```python
from build123d import *

# Parameters (mm, degrees)
SKETCH1_W           = 150
SKETCH1_H           = 30
BOSS_EXTRUDE1_DEPTH = 15
CUT_EXTRUDE1_DEPTH  = 5
SKETCH3_R           = 0.75
CUT_EXTRUDE2_DEPTH  = 30
CUT_EXTRUDE3_DEPTH  = 5


with BuildPart() as part:
    # Sketch1 → Boss-Extrude1 (new body)
    with BuildSketch(Plane(origin=(0, 0, 0), x_dir=(1, 0, 0), z_dir=(0, 1, 0))):
        with Locations((75, 15)):
            Rectangle(SKETCH1_W, SKETCH1_H)
    extrude(amount=BOSS_EXTRUDE1_DEPTH)

    # Sketch2 → Cut-Extrude1 (cut)
    with BuildSketch(Plane(origin=(0, 15, 0), x_dir=(1, 0, 0), z_dir=(0, 1, 0))):
        with BuildLine():
            Line((-20, 22.5), (20, 22.5))
            ThreePointArc((20, 22.5), (27.5, 15), (20, 7.5))
            Line((20, 7.5), (-20, 7.5))
            ThreePointArc((-20, 7.5), (-27.5, 15), (-20, 22.5))
        make_face()
        with BuildLine():
            Line((170, 22.5), (130, 22.5))
            ThreePointArc((130, 22.5), (122.5, 15), (130, 7.5))
            Line((130, 7.5), (170, 7.5))
            ThreePointArc((170, 7.5), (177.5, 15), (170, 22.5))
        make_face()
    extrude(amount=-CUT_EXTRUDE1_DEPTH, mode=Mode.SUBTRACT)

    # Sketch3 → Cut-Extrude2 (cut)
    with BuildSketch(Plane.XY):
        with Locations((25, 7.5)):
            Circle(SKETCH3_R)
        with Locations((75, 7.5)):
            Circle(SKETCH3_R)
        with Locations((125, 7.5)):
            Circle(SKETCH3_R)
    extrude(amount=-CUT_EXTRUDE2_DEPTH, mode=Mode.SUBTRACT)

    # Sketch4 → Cut-Extrude3 (cut)
    with BuildSketch(Plane(origin=(0, 15, 0), x_dir=(1, 0, 0), z_dir=(0, 1, 0))):
        with BuildLine():
            Line((37.5, 25), (112.5, 25))
            ThreePointArc((112.5, 25), (116.035533906, 23.535533906), (117.5, 20))
            Line((117.5, 20), (117.5, 10))
            ThreePointArc((117.5, 10), (116.035533906, 6.464466094), (112.5, 5))
            Line((112.5, 5), (37.5, 5))
            ThreePointArc((37.5, 5), (33.964466094, 6.464466094), (32.5, 10))
            Line((32.5, 10), (32.5, 20))
            ThreePointArc((32.5, 20), (33.964466094, 23.535533906), (37.5, 25))
        make_face()
    extrude(amount=-CUT_EXTRUDE3_DEPTH, mode=Mode.SUBTRACT)


solid = part.part
```
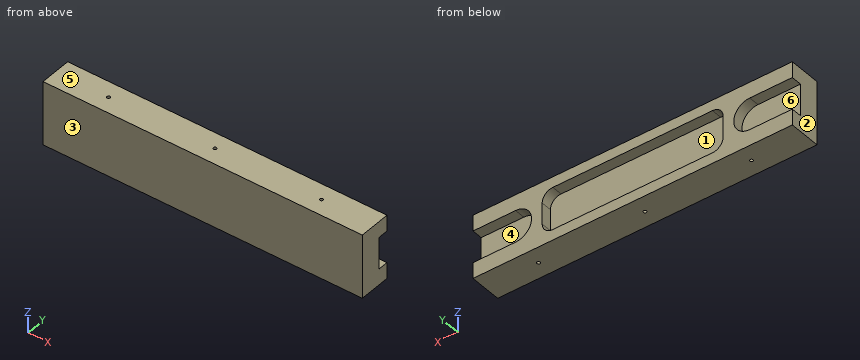
Verification items for the finished model (mm, model axes). Face numbers are marked on the shaded views. A direction names the side the tool comes from. Coordinates: 2 decimals unless noted, no trailing zeros. Write each loop counter-clockwise with the first axis right and the second up, starting at its lowest first coordinate (ties: lowest second). Pieces come first, ordered by that corner, then holes. Notation, with made-up numbers: M 20.25,31 L 72.25,31 A7 cw 72.25,38 Z; hole C 53,17.25 d11. An arc over 180 degrees is marked long. One line per item, written item: value.
Item 1: Access from +Z, -Z, +X, -X, +Y, -Y to the whole of each face (thin tool, end or side, straight path). Record for the marked faces 4, 5 and 6.
Check sheet entries:
face 4: +X, +Y
face 5: +Z, +X, -X, +Y, -Y
face 6: -X, +Y
Item 2: Scan lines: line 1 along Y through (x, z) = (25, -21.25); line 2 along X through (y, z) = (7.25, -22); line 3 along Y through (x, z) = (75, -16.75). Record each from-to range of solid material in increasing order.
Check sheet entries:
line 1: y = 0 to 6.75, 8.25 to 15
line 2: x = 0 to 24.29, 25.71 to 74.29, 75.71 to 124.29, 125.71 to 150
line 3: y = 0 to 6.75, 8.25 to 10
Item 3: Section check B-B, the plane z = -15. Record the boundary of the cut face in (x, y), plus the area to 3 significant figures.
Check sheet entries:
outline: M 0,0 L 150,0 L 150,10 L 122.5,10 L 122.5,15 L 117.5,15 L 117.5,10 L 32.5,10 L 32.5,15 L 27.5,15 L 27.5,10 L 0,10 Z; hole C 25,7.5 d1.5; hole C 75,7.5 d1.5; hole C 125,7.5 d1.5
area: 1,540 mm^2
Item 4: Mould release check, pull along X, two halves, no side actions. Record for the marked faces 1, 2 and 3: pulls with the +X half, pulls with the -X half, needs draft (parallel to the pull), parting line crosses it, or undercut.
Check sheet entries:
face 1: undercut
face 2: pulls with the -X half
face 3: needs draft
Item 5: Gauge pin test, flat ends, axial feed: pin 1 Ø2.5 at (y, z) = (13, -17) entering from +X; pin 2 Ø1.5 at (y, z) = (12, -14.5) entering from -X; pin 3 Ø12 at (x, z) = (138.5, -14.5) entering from +Y; pin 4 Ø1.2 at (x, y) = (125, 7.5) entering from +Z. Record the tip position at first contact, or that the pin passes through.
Check sheet entries:
pin 1: stops at x = 123.24
pin 2: stops at x = 27.4
pin 3: stops at y = 10
pin 4: passes through
Item 6: Section check A-A, the plane y = 13.75. Record the boundary of the cut face in (x, z), plus the area to 3 significant figures.
Check sheet entries:
outline: M 0,-30 L 150,-30 L 150,-22.5 L 130,-22.5 A7.5 cw 130,-7.5 L 150,-7.5 L 150,0 L 0,0 L 0,-7.5 L 20,-7.5 A7.5 cw 20,-22.5 L 0,-22.5 Z; hole M 32.5,-20 A5 ccw 37.5,-25 L 112.5,-25 A5 ccw 117.5,-20 L 117.5,-10 A5 ccw 112.5,-5 L 37.5,-5 A5 ccw 32.5,-10 Z
area: 2,040 mm^2
